Verification items for the finished model (mm, model axes). Give positions to 0.01 mm unless a question says otherwise; leave off trailing zeros. Write each loop counter-clockwise with the first axis right and the second up, starting at its lowest first coordinate (ties: lowest second). Pieces come first, ordered by that corner, then holes.
from build123d import *

# Parameters (mm, degrees)
SKETCH1_W           = 140
SKETCH1_H           = 165
SKETCH1_R           = 2.075495439
SKETCH1_R_2         = 1.55
SKETCH1_R_3         = 1.99999854
SKETCH1_W_2         = 3
SKETCH1_H_2         = 3
SKETCH1_W_3         = 3.071243945
SKETCH1_H_3         = 25.44744983
SKETCH1_W_4         = 2.90164108
SKETCH1_H_4         = 23.501913203
BOSS_EXTRUDE1_DEPTH = 3


with BuildPart() as part:
    # Sketch1 → Boss-Extrude1 (new body)
    with BuildSketch(Plane(origin=(0, 0, 0), x_dir=(1, 0, 0), z_dir=(0, 1, 0))):
        Rectangle(SKETCH1_W, SKETCH1_H)
        with Locations(Location((0, 78.220695367, 0), (0, 0, 270))):
            Circle(SKETCH1_R, mode=Mode.SUBTRACT)
        with Locations(Location((-44.593659723, -20.900034899, 0), (0, 0, 270))):
            Circle(SKETCH1_R_2, mode=Mode.SUBTRACT)
        with Locations(Location((44.593659723, -20.900034899, 0), (0, 0, 270))):
            Circle(SKETCH1_R_2, mode=Mode.SUBTRACT)
        with Locations(Location((-58.3565, 13.925245662, 0), (0, 0, 270))):
            Circle(SKETCH1_R_3, mode=Mode.SUBTRACT)
        with Locations(Location((-58.3565, 64.407745662, 0), (0, 0, 270))):
            Circle(SKETCH1_R_3, mode=Mode.SUBTRACT)
        with Locations(Location((57.531, 64.407745662, 0), (0, 0, 270))):
            Circle(SKETCH1_R_3, mode=Mode.SUBTRACT)
        with Locations(Location((57.531, 13.925245662, 0), (0, 0, 270))):
            Circle(SKETCH1_R_3, mode=Mode.SUBTRACT)
        with Locations((-23.843659723, -1.031919399)):
            Rectangle(SKETCH1_W_2, SKETCH1_H_2, mode=Mode.SUBTRACT)
        with Locations((-64.843659723, -1.031884133)):
            Rectangle(SKETCH1_W_2, SKETCH1_H_2, mode=Mode.SUBTRACT)
        with Locations((-64.843659723, -57.768115133)):
            Rectangle(SKETCH1_W_2, SKETCH1_H_2, mode=Mode.SUBTRACT)
        with Locations((-43.843659723, -57.768150399)):
            Rectangle(SKETCH1_W_2, SKETCH1_H_2, mode=Mode.SUBTRACT)
        with Locations((-43.843659723, -34.531919899)):
            Rectangle(SKETCH1_W_2, SKETCH1_H_2, mode=Mode.SUBTRACT)
        with Locations((-23.843659723, -27.268149899)):
            Rectangle(SKETCH1_W_2, SKETCH1_H_2, mode=Mode.SUBTRACT)
        with Locations((43.843659723, -34.531919899)):
            Rectangle(SKETCH1_W_2, SKETCH1_H_2, mode=Mode.SUBTRACT)
        with Locations((23.843659723, -27.268149899)):
            Rectangle(SKETCH1_W_2, SKETCH1_H_2, mode=Mode.SUBTRACT)
        with Locations((43.843659723, -57.768150399)):
            Rectangle(SKETCH1_W_2, SKETCH1_H_2, mode=Mode.SUBTRACT)
        with Locations((64.843659723, -57.768115133)):
            Rectangle(SKETCH1_W_2, SKETCH1_H_2, mode=Mode.SUBTRACT)
        with Locations((64.843659723, -1.031884133)):
            Rectangle(SKETCH1_W_2, SKETCH1_H_2, mode=Mode.SUBTRACT)
        with Locations((23.843659723, -1.031919399)):
            Rectangle(SKETCH1_W_2, SKETCH1_H_2, mode=Mode.SUBTRACT)
        with Locations((-35.561590823, -58.032613537)):
            Rectangle(SKETCH1_W_3, SKETCH1_H_3, mode=Mode.SUBTRACT)
        with Locations((34.92934681, -59.005381851)):
            Rectangle(SKETCH1_W_4, SKETCH1_H_4, mode=Mode.SUBTRACT)
    extrude(amount=BOSS_EXTRUDE1_DEPTH)


solid = part.part
Item 1: Release check for a two-part mould opening along Z. For faces 1 (the face through (-1, 0, -1)), 2 (the face through (0.091, 1.479, -80.294)), 3 (the face through (59.514, 1.479, -14.186)) record: released by +Z, released by -Z, zero draft, split by the parting line, or undercut.
Answer key:
face 1: zero draft
face 2: undercut
face 3: undercut
Item 2: Sectioned sample at A-A on x = 0. Record the cut outline in (y, z), then the cut area to 3 significant figures.
Answer key:
outline: (0, -82.5) - (3, -82.5) - (3, -80.3) - (0, -80.3) - close; (0, -76.15) - (3, -76.15) - (3, 82.5) - (0, 82.5) - close
area: 483 mm2
Item 3: Scan lines: line 1 along Z through (x, y) = (-23, 1.65); line 2 along X through (y, z) = (2, 27); line 3 along X through (y, z) = (2.25, 55). Record each from-to range of solid material in increasing order.
Answer key:
line 1: z = -82.5 to -0.47, 2.53 to 25.77, 28.77 to 82.5
line 2: x = -70 to -25.34, -22.34 to 22.34, 25.34 to 70
line 3: x = -70 to -37.1, -34.03 to 33.48, 36.38 to 70
